```python
from build123d import *

# Parameters (mm, degrees)
SKETCH_1_R          = 1.55
EXTRUDE_1_DEPTH     = 2
FILLET_1_R          = 3
FILLET_2_R          = 0.2
SKETCH_3_R          = 0.75
CUT_EXTRUDE_1_DEPTH = 1


with BuildPart() as part:
    # 草图1 → 凸台-拉伸1 (new body)
    with BuildSketch(Plane(origin=(0, 0, 0), x_dir=(1, 0, 0), z_dir=(0, 1, 0))):
        with BuildLine():
            Line((-9.427629845, 12.118007633), (-14.205972572, 5.57250637))
            ThreePointArc((-14.205972572, 5.57250637), (-13.333741258, -0.01669863), (-7.744536258, 0.855532684))
            Line((-7.744536258, 0.855532684), (-2.966193531, 7.401033946))
            ThreePointArc((-2.966193531, 7.401033946), (2.156455687, 5.844533995), (7.508476858, 5.702771934))
            Line((7.508476858, 5.702771934), (9.973957748, -2.017173013))
            ThreePointArc((9.973957748, -2.017173013), (15.001264118, -4.610663069), (17.594754173, 0.416643301))
            Line((17.594754173, 0.416643301), (15.129273283, 8.136588247))
            Line((15.129273283, 8.136588247), (19.53886034, 20.548398832))
            ThreePointArc((19.53886034, 20.548398832), (2.94865648, 10.730730666), (-9.689752685, 25.287244194))
            Line((-9.689752685, 25.287244194), (-9.427629845, 12.118007633))
        make_face()
        with Locations(Location((13.784355961, -0.800264856, 0), (0, 0, 270))):
            Circle(SKETCH_1_R, mode=Mode.SUBTRACT)
        with Locations(Location((-10.975254415, 3.214019527, 0), (0, 0, 270))):
            Circle(SKETCH_1_R, mode=Mode.SUBTRACT)
    extrude(amount=EXTRUDE_1_DEPTH)

    # 圆角1
    fillet_1_edges = [part.edges().sort_by_distance(p)[0] for p in [
        (-9.427629845, 1, -12.118007633),
        (15.129273283, 1, -8.136588247),
        (7.508476858, 1, -5.702771934),
        (-2.966193531, 1, -7.401033946),
    ]]
    fillet(fillet_1_edges, radius=FILLET_1_R)

    # 草图2 → 切除-旋转1 (revolve, cut)
    with BuildSketch(Plane(origin=(5.357266973, 0, 0), x_dir=(0, -1, 0), z_dir=(-1, 0, 0))):
        with BuildLine():
            Line((5.030031962, -25.586742765), (-45.030031962, -25.586742765))
            ThreePointArc((-45.030031962, -25.586742765), (-20, -0.556710804), (5.030031962, -25.586742765))
        make_face()
    revolve(axis=Axis((5.357266973, -5.030031962, -25.586742765), (0, 1, 0)), mode=Mode.SUBTRACT)

    # 圆角2
    # the kernel refuses this fillet: 0.2 mm, written as the material it takes off along each edge
    with BuildSketch(Plane(origin=(19.53886034, 20, -20.548398832), x_dir=(0.01660114178813642, -0.9987697013737693, -0.04672778305335893), z_dir=(0.33436181166525863, 0.049589148185380114, -0.9411392539269492))) as fillet_2_piece_1:
        with BuildLine():
            CenterArc((20.396862817, 0.2), FILLET_2_R, 143.943391902, 126.056608098)
            ThreePointArc((20.235175643, 0.317716854), (20.118215024, 0.158394169), (20, 0))
            Line((20, 0), (20.396862817, 0))
        make_face()
    revolve(axis=Axis((19.53886034, 20, -20.548398832), (-0.9422985625539585, 0, -0.3347736832678813)), revolution_arc=31.526762102, mode=Mode.SUBTRACT)
    with BuildSketch(Plane(origin=(-9.689752685, 20, -25.287244194), x_dir=(0.009551792559497672, -0.8772773226727593, 0.4798888021021284), z_dir=(0.017458026871632594, 0.4799838529826972, 0.87710359603278))) as fillet_2_piece_2:
        with BuildLine():
            CenterArc((20.396862817, 0.2), FILLET_2_R, 143.943391902, 126.056608098)
            ThreePointArc((20.235175643, 0.317716854), (20.118215024, 0.158394169), (20, 0))
            Line((20, 0), (20.396862817, 0))
        make_face()
    revolve(axis=Axis((-9.689752685, 20, -25.287244194), (0.9998019706705172, 0, -0.019900237268694068)), revolution_arc=31.526762102, mode=Mode.SUBTRACT)
    with BuildSketch(Plane(origin=(5.357266973, 2, -25.586742765), x_dir=(0.6563745928876489, 0, 0.7544351488442022), z_dir=(0.7544351488442022, 0, -0.6563745928876489))) as fillet_2_piece_3:
        with BuildLine():
            CenterArc((17.473251351, 0.2), FILLET_2_R, 226.167089334, 43.832910666)
            Line((17.473251351, 0), (17.392599001, 0))
            ThreePointArc((17.392599001, 0), (17.363691769, 0.027886958), (17.334739824, 0.055727492))
        make_face()
    revolve(axis=Axis((5.357266973, 2, -25.586742765), (0, -1, 0)), revolution_arc=100.466423908, mode=Mode.SUBTRACT)

    # 草图3 → 切除-拉伸1 (cut)
    with BuildSketch(Plane.XZ):
        with Locations(Location((-8.027145861, -7.252417223, 0), (0, 0, 270))):
            Circle(SKETCH_3_R)
    extrude(amount=-CUT_EXTRUDE_1_DEPTH, mode=Mode.SUBTRACT)


solid = part.part
```
Here's how the part is built. I have some questions about the finished solid (model axes, mm). A direction names the side the tool comes from. Give positions to 0.01 mm unless a question says otherwise; leave off trailing zeros. Loops run counter-clockwise (first coordinate to the right, second up) from the corner with the lowest first, then second, coordinate; pieces in that order, holes last. Notation, with made-up numbers: M 83,83 L 126,83 A30 ccw 126,119 Z; hole C -12,24.5 d2. An arc over 180 degrees is marked long. Use one line per item in the form item = value. Start each with the question number.
Q1. Thinking about a two-plate mould opening in Z: for faces 1 (the cylindrical face through (12.271, 0.986, 0.464)), 2 (the flat face through (9.08, 0.99, -0.78)), 3 (the cylindrical face through (-8.69, 0.49, -7.6)), 4 (the cylindrical face through (-13.404, 0.986, -0.036)), which applies, +Z half, -Z half, draft (parallel to the pull), parting line (faces both ways), or undercut?
Q2. I need wall thicknesses on line 1 along X through (y, z) = (0.2, -3.75); line 2 along X through (y, z) = (0.55, -12); line 3 along Z through (x, y) = (1.5, 0.7). Which ranges of each line are inside material? Lowest first, please.
Q3. If we section it at D-D (x = -13): Write out the boundary of the cut face in (y, z), then the cut area to 3 significant figures.
Q4. Which directions (+Z, -Z, +X, -X, +Y, -Y) give clear straight access to the entire face, cutting with the end or side of a thin tool? Please do faces 5 (the flat face through (-8, 1, -7)), 6 (the flat face through (16.53, 0.99, -3.75)), 7 (the cylindrical face through (2.112, 0.986, -5.852)).
Q5. If we section it at C-C (y = 0.55): State how many separate pieces and enclosed holes the cut face has, then the cut area to 3 significant figures.
Q6. If we section it at A-A (z = 1.5): Write out the boundary of the cut face in (x, y).
Q7. If we section it at B-B (z = -1.25): Write out the boundary of the cut face in (x, y).
Q8. Will these pins go through, and if not, where does the flat tip stop? pin 1 Ø6 at (x, z) = (2, -0.5) entering from +Y; pin 2 Ø1 at (y, z) = (1, -18.5) entering from -X; pin 3 Ø4 at (x, z) = (13.78, 0.8) entering from +Y.
Taken from the geometry:
q1.face_1 = undercut
q1.face_2 = +Z half
q1.face_3 = undercut
q1.face_4 = parting line
q2.line_1 = -14.94 to -12.43, -9.52 to -5.63, 8.12 to 16.53
q2.line_2 = -9.64 to -2.62, 13.33 to 16.5
q2.line_3 = -10.12 to -5.96
q3.outline = M 0,-7.22 L 2,-7.22 L 2,0.24 L 0,0.24 Z
q3.area = 14.9 mm^2
q4.face_5 = -Y
q4.face_6 = +X, +Y, -Y
q4.face_7 = +Z, +Y, -Y
q5.separate_pieces = 1
q5.enclosed_holes = 3
q5.area = 287 mm^2
q6.outline = M 9.81,0 L 12.4,0 L 12.4,2 L 9.81,2 Z; M 15.17,0 L 17.72,0 L 17.72,2 L 15.17,2 Z
q7.outline = M -14.46,0 L -7.46,0 L -7.46,2 L -14.46,2 Z; M 8.93,0 L 17.33,0 L 17.33,2 L 8.93,2 Z
q8.pin_1 = through
q8.pin_2 = -9.56
q8.pin_3 = 2
